```python
from build123d import *
from build123d import SkipClean  # not in build123d's __all__

# Parameters (mm, degrees)
F0_W      = 50.8
F0_H      = 31.75
F1_DEPTH  = 6.35
F2_R      = 3.175
F3_DEPTH  = 6.35
F4_W      = 50.8
F4_H      = 12.7
F5_DEPTH  = 57.15
F7_DEPTH  = 12.7
F8_DEPTH  = 12.7
F9_R      = 6.35
F10_DEPTH = 38.1


with BuildPart() as f1:
    # F0 (on Top) → F1 (new body)
    with BuildSketch(Plane.XY):
        with Locations((25.4, 15.875)):
            Rectangle(F0_W, F0_H)
    extrude(amount=F1_DEPTH)

    # F2 (on face) → F3 (cut)
    with BuildSketch(Plane.XY.offset(6.35)):
        with Locations((41.275, 9.525)):
            Circle(F2_R)
        with Locations((9.525, 9.525)):
            Circle(F2_R)
        with BuildLine():
            ThreePointArc((9.525, 0), (3.3956264222, 3.3956264222), (0, 9.525))
            Line((0, 9.525), (0, 0))
            Line((0, 0), (9.525, 0))
        make_face()
        with BuildLine():
            ThreePointArc((50.8, 9.525), (47.4043735778, 3.3956264222), (41.275, 0))
            Line((41.275, 0), (50.8, 0))
            Line((50.8, 0), (50.8, 9.525))
        make_face()
    extrude(amount=-F3_DEPTH, mode=Mode.SUBTRACT)

    # F4 (on face) → F5 (join)
    with BuildSketch(Plane.XY.offset(6.35)):
        with Locations((25.4, 25.4)):
            Rectangle(F4_W, F4_H)
    extrude(amount=F5_DEPTH)

    # F6 (on face) → F7 (cut)
    with BuildSketch(Plane.XZ.offset(-19.05)):
        with BuildLine():
            ThreePointArc((12.7, 44.45), (25.4, 57.15), (38.1, 44.45))
            Line((38.1, 44.45), (38.1, 19.05))
            ThreePointArc((38.1, 19.05), (41.8197438789, 10.0697438789), (50.8, 6.35))
            Line((50.8, 6.35), (50.8, 63.5))
            Line((50.8, 63.5), (0, 63.5))
            Line((0, 63.5), (0, 6.35))
            ThreePointArc((0, 6.35), (8.9802561211, 10.0697438789), (12.7, 19.05))
            Line((12.7, 19.05), (12.7, 44.45))
        make_face()
    extrude(amount=-F7_DEPTH, mode=Mode.SUBTRACT)

    # F6 (on face) → F8 (join)
    with BuildSketch(Plane.XZ.offset(-19.05)):
        with BuildLine():
            ThreePointArc((12.7, 44.45), (25.4, 31.75), (38.1, 44.45))
            ThreePointArc((38.1, 44.45), (25.4, 57.15), (12.7, 44.45))
        make_face()
    with SkipClean():  # cleaning this boolean's faces spoils the solid; the shape is the same uncleaned
        extrude(amount=F8_DEPTH)

    # F9 (on face) → F10 (cut)
    with BuildSketch(Plane.XZ.offset(-6.35)):
        with Locations((25.4, 44.45)):
            Circle(F9_R)
    with SkipClean():  # cleaning this boolean's faces spoils the solid; the shape is the same uncleaned
        extrude(amount=-F10_DEPTH, mode=Mode.SUBTRACT)


solid = f1.part
```
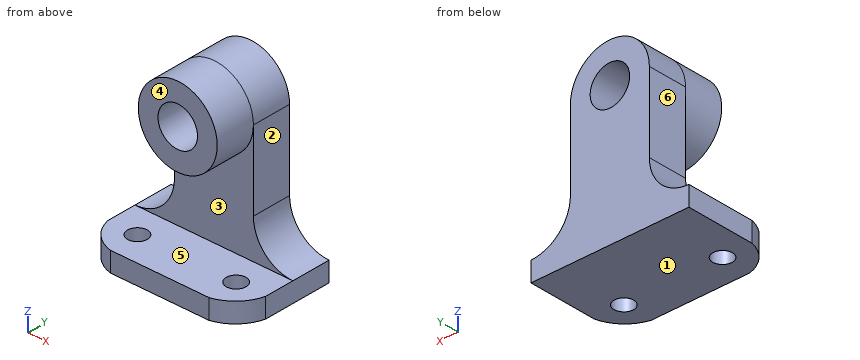
The model under review builds one solid part; all positions refer to its coordinate system, in mm. Face numbers are marked on the shaded views. A direction names the side the tool comes from. Round coordinates to 2 decimals unless told otherwise and drop trailing zeros. Loops run counter-clockwise (first coordinate to the right, second up) from the corner with the lowest first, then second, coordinate; pieces in that order, holes last. Notation, with made-up numbers: (52.5, -22.5) - (72.5, -22.5) arc R33 cw to (72.5, 12.5) - close; hole circle Ø4 at (-18.5, -15.5). An arc over 180 degrees is marked (long way). Write each question's results on one line, items separated by ' | '. Start each with the question number.
Q1. Take a section at D-D on y = 7.5. Give the boundary of the cut face in (x, z).
Q2. Take a section at B-B on x = 25.4. Give the boundary of the cut face in (y, z), plus the area to 3 significant figures.
Q3. Tool access review of the marked faces 4, 5 and 6: name each direction out of +Z, -Z, +X, -X, +Y, -Y from which nothing blocks a thin tool from reaching the whole face with its end or side.
Q4. Wall thickness on line 1 along X through (y, z) = (6.5, 44.5); line 2 along Z through (x, y) = (25, 19); line 3 along Z through (x, y) = (46, 17.5): over which ranges is each line inside the solid? List them lowest first. Write a range as [from, to].
Q5. Insertion check: P1, Ø7.5, axis at x = 21.5, z = 43, coming from the -Y side; P2, Ø12, axis at y = 7.5, z = 30, coming from the +X side; P3, Ø6.5, axis at y = 25.5, z = 26.5, coming from the -X side. Each pin has a flat end and moves straight along its axis. Give the tip position at first contact, or say it passes through.
Q6. Draft analysis for pull direction Z (two halves, no side actions). For the marked faces 1, 2 and 3, state which applies: pulls with the +Z half, pulls with the -Z half, needs draft (parallel to the pull), parting line crosses it, or undercut.
Q7. Take a section at A-A on y = 16.5. Give the boundary of the cut face in (x, z), plus the area to 3 significant figures.
Q8. Take a section at C-C on z = 49. Give the boundary of the cut face in (x, y), plus the area to 3 significant figures.
Data:
1) outline: (0.65, 0) - (7.08, 0) - (7.08, 6.35) - (0.65, 6.35) - close; (11.97, 0) - (38.83, 0) - (38.83, 6.35) - (11.97, 6.35) - close; circle Ø25.4 at (25.4, 44.45); (43.72, 0) - (50.15, 0) - (50.15, 6.35) - (43.72, 6.35) - close; hole circle Ø12.7 at (25.4, 44.45)
2) outline: (0, 0) - (31.75, 0) - (31.75, 38.1) - (6.35, 38.1) - (6.35, 31.75) - (19.05, 31.75) - (19.05, 6.35) - (0, 6.35) - close; (6.35, 50.8) - (31.75, 50.8) - (31.75, 57.15) - (6.35, 57.15) - close | area: 847 mm²
3) face 4: +Z, +X, -X, -Y | face 5: +X, -X, -Y | face 6: +Z, -X, +Y, -Y
4) line 1: x = [12.7, 19.05], [31.75, 38.1] | line 2: z = [0, 6.35], [31.76, 38.11], [50.79, 57.14] | line 3: z = [0, 6.35]
5) P1: stops at y = 6.35 | P2: stops at x = 34.88 | P3: stops at x = 12.7
6) face 1: pulls with the -Z half | face 2: needs draft | face 3: undercut
7) outline: (0, 0) - (50.8, 0) - (50.8, 6.35) - (0, 6.35) - close; circle Ø25.4 at (25.4, 44.45); hole circle Ø12.7 at (25.4, 44.45) | area: 703 mm²
8) outline: (13.54, 6.35) - (20.97, 6.35) - (20.97, 31.75) - (13.54, 31.75) - close; (29.83, 6.35) - (37.26, 6.35) - (37.26, 31.75) - (29.83, 31.75) - close | area: 377 mm²
